Verification items for the finished model (mm, model axes). A direction names the side the tool comes from. Round coordinates to 2 decimals unless told otherwise and drop trailing zeros. Loops run counter-clockwise (first coordinate to the right, second up) from the corner with the lowest first, then second, coordinate; pieces in that order, holes last. Notation, with made-up numbers: M -11.75,61.5 L 3.25,61.5 A22 cw 3.25,78.5 Z; hole C -17.75,-6 d4. An arc over 180 degrees is marked long. Write item = value, one per line. Start each with the question number.
from build123d import *

# Parameters (mm, degrees)
F0_W     = 25.4
F0_H     = 7.874
F0_H_2   = 4.826
F0_H_3   = 19.05
F1_DEPTH = 25.4


with BuildPart() as f1:
    # F0 (on Front) → F1 (new body)
    with BuildSketch(Plane.XZ):
        with BuildLine():
            ThreePointArc((49.149, 61.849), (48.2646519361, 61.8344723936), (47.3812582222, 61.790905252))
            add(Edge.make_bspline(
                [(47.3812582222, 61.790905252), (47.9669561988, 61.8111847616), (48.5561975061, 61.8305479146), (49.149, 61.849)],
                knots=[103.5782893444, 103.5782893444, 103.5782893444, 103.5782893444, 104.4715308206, 104.4715308206, 104.4715308206, 104.4715308206], degree=3))
        make_face()
        with BuildLine():
            Line((-41.275, 9.525), (22.225, 9.525))
            Line((22.225, 9.525), (22.225, 34.925))
            ThreePointArc((22.225, 34.925), (29.4958010794, 53.3275418947), (47.3812582222, 61.790905252))
            add(Edge.make_bspline(
                [(-41.275, 9.525), (-40.8068549943, 44.7662530835), (-20.5349728413, 59.4393385436), (47.3812582222, 61.790905252)],
                knots=[0, 0, 0, 0, 103.5782893444, 103.5782893444, 103.5782893444, 103.5782893444], degree=3))
        make_face()
        with Locations((73.025, 38.862)):
            Rectangle(F0_W, F0_H)
        with Locations((73.025, 64.262)):
            Rectangle(F0_W, F0_H_2)
        Polygon((85.725, 61.849), (85.725, 42.799), (85.725, 34.925), (111.125, 34.925), (111.125, 66.675), (85.725, 66.675), align=None)
        with BuildLine():
            Line((22.225, 9.525), (41.275, 9.525))
            Line((41.275, 9.525), (41.275, 34.925))
            ThreePointArc((41.275, 34.925), (43.5812412049, 40.4927587951), (49.149, 42.799))
            Line((49.149, 42.799), (60.325, 42.799))
            Line((60.325, 42.799), (60.325, 61.849))
            Line((60.325, 61.849), (49.149, 61.849))
            add(Edge.make_bspline(
                [(47.3812582222, 61.790905252), (47.9669561988, 61.8111847616), (48.5561975061, 61.8305479146), (49.149, 61.849)],
                knots=[103.5782893444, 103.5782893444, 103.5782893444, 103.5782893444, 104.4715308206, 104.4715308206, 104.4715308206, 104.4715308206], degree=3))
            ThreePointArc((47.3812582222, 61.790905252), (29.4958010794, 53.3275418947), (22.225, 34.925))
            Line((22.225, 34.925), (22.225, 9.525))
        make_face()
        with Locations((73.025, 52.324)):
            Rectangle(F0_W, F0_H_3)
    extrude(amount=F1_DEPTH)


solid = f1.part
1. Thickness scan on line 1 (Z direction, x = 57, y = -19.75); line 2 (Z direction, x = 97, y = -23.75) (3 decimals); line 3 (X direction, y = -20.25, z = 42) (3 decimals). Record the ranges inside material, lowest first.
2. Gauge pin test, flat ends, axial feed: P1, Ø1, axis at y = -6.5, z = 27, coming from the -X side; P2, Ø4, axis at y = -7, z = 37, coming from the -X side; P3, Ø8, axis at y = -13, z = 41.5, coming from the -X side; P4, Ø2, axis at x = 10, z = 54, coming from the +Y side. Record the tip position at first contact, or that the pin passes through.
3. Mould release check, pull along X, two halves, no side actions. Record for faces 6 (the flat face through (111.125, -13, 51)), 7 (the flat face through (55, -13, 42.799)), 8 (the flat face through (34, -25.4, 39)), 9 (the flat face through (60.325, -13, 39)): pulls with the +X half, pulls with the -X half, needs draft (parallel to the pull), parting line crosses it, or undercut.
4. Section check B-B, the plane x = 56.5. Enter the section's corners in (y, z), and give its area (3 significant figures).
5. Section check A-A, the plane x = 76. Enter the section's corners in (y, z) (3 decimals).
6. Tool access check on faces 1 (the flat face through (34, 0, 39)), 2 (the flat face through (60.325, -13, 64)), 3 (the flat face through (85, -13, 34.925)), 4 (the cylindrical face through (43.52, -12.52, 40.43)), 5 (the flat face through (86, -13, 66.675)). Record the directions out of +Z, -Z, +X, -X, +Y, -Y that give a thin tool (end or side, any length) a straight path to the whole face; none if there is none.
Computed values:
q1.line_1 = 42.8 to 61.85
q1.line_2 = 34.925 to 66.675
q1.line_3 = -29.902 to 45.693, 60.325 to 111.125
q2.P1 = -38.97
q2.P2 = -35.31
q2.P3 = -33.69
q2.P4 = 0
q3.face_6 = pulls with the +X half
q3.face_7 = undercut
q3.face_8 = needs draft
q3.face_9 = undercut
q4.outline = M -25.4,42.8 L 0,42.8 L 0,61.85 L -25.4,61.85 Z
q4.area = 484 mm2
q5.outline = M -25.4,34.925 L 0,34.925 L 0,66.675 L -25.4,66.675 Z
q6.face_1 = +Z, -Z, +X, -X, +Y
q6.face_2 = +Z, -X, +Y, -Y
q6.face_3 = -Z, +X, +Y, -Y
q6.face_4 = -Z, +Y, -Y
q6.face_5 = +Z, +X, -X, +Y, -Y
